Input: part model. Units: mm. Frame: model coordinates. Round coordinates to 2 decimals unless told otherwise and drop trailing zeros. Loops run counter-clockwise (first coordinate to the right, second up) from the corner with the lowest first, then second, coordinate; pieces in that order, holes last. Notation, with made-up numbers: (2.5, 81) - (36.5, 81) arc R16 cw to (36.5, 108) - close; hole circle Ø6 at (79.25, 30). An arc over 180 degrees is marked (long way). One line per question, with ' | ' between items. Start each with the question number.
Item 1: First-contact query: pin 1 (1 mm diameter, centred on y = 29, z = 3.5, fed in from +X); pin 2 (2 mm diameter, centred on y = -17.5, z = 1, fed in from -X). Flat tips, straight axial feed; report the tip coordinate or a pass-through.
Item 2: Section D-D, the plane x = 49.5. Return loops of the section in (y, z).
Item 3: Draft query along Y for faces 1 (the face through (-10.731, -8.578, 1.972)), 2 (the face through (-59.94, -2.64, 1.97)), 3 (the face through (-1, -12, 4)). Return one class per face: pulls with the +Y half, pulls with the -Y half, needs draft (parallel to the pull), parting line crosses it, or undercut.
Item 4: Section C-C, the plane y = -25.5. Return loops of the section in (x, z).
Item 5: Section A-A, the plane x = 0. Return loops of the section in (y, z), plus the area to 3 significant figures.
Item 6: Section B-B, the plane z = 0.65. Return loops of the section in (x, y).
Item 7: Material intervals for line 1 along Y through (x, z) = (0, 1.55); line 2 along X through (y, z) = (1, 2.25); line 3 along X through (y, z) = (10.5, 0.35), sorted ascending.
Autodesk Inventor part; units mm, degrees
ref_plane "YZ Plane" through (0, 0, 0) normal (1, 0, 0) x (0, 1, 0)
ref_plane "XZ Plane" through (0, 0, 0) normal (0, 1, 0) x (-1, 0, 0)
ref_plane "XY Plane" through (0, 0, 0) normal (0, 0, 1) x (1, 0, 0)
sketch "Эскиз1" plane through (0, 0, 0) normal (0, 0, 1) x (1, 0, 0)
  circle A0 centre (0, 0) radius 5
  circle A1 centre (0, 0) radius 60
  line L0 (0, -84) -> (0, 84) construction
  circle A2 centre (0, 0) radius 20.7 construction
  circle A3 centre (0, 12) radius 2.6
  line L1 (-84, 0) -> (84, 0) construction
  circle A4 centre (-10.3923, -6) radius 2.6
  circle A5 centre (10.3923, -6) radius 2.6
  dimension "d0" = 10
  dimension "d1" = 120
  dimension "d4" = 41.4
  dimension "d5" = 5.2
  dimension "d6" = 12
  dimension "d9" = 360
extrude "Выдавливание1" add sketch "Эскиз1" along normal blind 4
properties part number "Бортик конусной катушки"
Return value:
1) pin 1: x = 52.8 | pin 2: x = -57.69
2) outline: (-33.91, 0) - (33.91, 0) - (33.91, 4) - (-33.91, 4) - close
3) face 1: undercut | face 2: parting line crosses it | face 3: needs draft
4) outline: (-54.31, 0) - (54.31, 0) - (54.31, 4) - (-54.31, 4) - close
5) outline: (-60, 0) - (-5, 0) - (-5, 4) - (-60, 4) - close; (5, 0) - (9.4, 0) - (9.4, 4) - (5, 4) - close; (14.6, 0) - (60, 0) - (60, 4) - (14.6, 4) - close | area: 419 mm2
6) outline: circle Ø120 at (0, 0); hole circle Ø5.2 at (-10.39, -6); hole circle Ø10 at (0, 0); hole circle Ø5.2 at (0, 12); hole circle Ø5.2 at (10.39, -6)
7) line 1: -60 to -5, 5 to 9.4, 14.6 to 60 | line 2: -59.99 to -4.9, 4.9 to 59.99 | line 3: -59.07 to -2.12, 2.12 to 59.07
